CAD build for the part. Positions are in the model's coordinates, mm. Face numbers are marked on the shaded views. A direction names the side the tool comes from. Give positions to 0.01 mm unless a question says otherwise; leave off trailing zeros. Write each loop counter-clockwise with the first axis right and the second up, starting at its lowest first coordinate (ties: lowest second). Pieces come first, ordered by that corner, then holes. Notation, with made-up numbers: (71.25, 51.25) - (75.25, 51.25) arc R13 cw to (75.25, 58.25) - close; hole circle Ø10 at (51.25, -19.5). An arc over 180 degrees is marked (long way). Write item = value, one per line. Start each with the question number.
```python
from build123d import *

# Parameters (mm, degrees)
SKETCH1_W           = 85.95
SKETCH1_H           = 85.95
BOSS_EXTRUDE1_DEPTH = 85.95
SKETCH2_W           = 83.95
SKETCH2_H           = 83.95
CUT_EXTRUDE1_DEPTH  = 83.95
CAVITY1_OUTLINE_R   = 13
CAVITY1_DEPTH       = 2
CAVITY2_OUTLINE_R   = 13
CAVITY2_DEPTH       = 2
CAVITY4_START       = -85.95
CAVITY4_OUTLINE_R   = 13
CAVITY4_DEPTH       = 2
CUT_EXTRUDE3_DEPTH  = 148.724092483
BOSS_EXTRUDE2_DEPTH = 2
CUT_EXTRUDE4_REACH  = 150.87
SKETCH8_W           = 2
SKETCH8_H           = 63.308692683
CUT_EXTRUDE5_REACH  = 150.87
SKETCH9_W           = 67.031257487
SKETCH9_H           = 2
CUT_EXTRUDE6_START  = -2
SKETCH10_W          = 2
SKETCH10_H          = 63.308692683
CUT_EXTRUDE6_DEPTH  = 2


# Read off the part's stored shape, not the designer's step: Cavity1, Cavity2, Cavity4
with BuildPart() as part:
    # Sketch1 → Boss-Extrude1 (new body)
    with BuildSketch(Plane.XY):
        with Locations((42.975, -42.975)):
            Rectangle(SKETCH1_W, SKETCH1_H)
    extrude(amount=BOSS_EXTRUDE1_DEPTH)

    # Sketch2 → Cut-Extrude1 (cut)
    with BuildSketch(Plane(origin=(0, 0, 0), x_dir=(1, 0, 0), z_dir=(0, 1, 0))):
        with Locations((43.975, -43.975)):
            Rectangle(SKETCH2_W, SKETCH2_H)
    extrude(amount=-CUT_EXTRUDE1_DEPTH, mode=Mode.SUBTRACT)

    # Cavity1 outline → Cavity1 (cut)
    with BuildSketch(Plane.XY):
        with Locations((38.75, -47.2)):
            Circle(CAVITY1_OUTLINE_R)
    extrude(amount=CAVITY1_DEPTH, mode=Mode.SUBTRACT)

    # Cavity2 outline → Cavity2 (cut)
    with BuildSketch(Plane.YZ):
        with Locations((-47.2, 39.55)):
            Circle(CAVITY2_OUTLINE_R)
    extrude(amount=CAVITY2_DEPTH, mode=Mode.SUBTRACT)

    # Cavity4 outline → Cavity4 (cut)
    with BuildSketch(Plane(origin=(0, 0, 0), x_dir=(1, 0, 0), z_dir=(0, 1, 0)).offset(CAVITY4_START)):
        with Locations((38.75, -39.55)):
            Circle(CAVITY4_OUTLINE_R)
    extrude(amount=CAVITY4_DEPTH, mode=Mode.SUBTRACT)

    # Sketch4 → Cut-Extrude3 (cut, through all)
    with BuildSketch(Plane.XY.offset(2)):
        Polygon((46.786231243, -31.127537514), (77.913768757, 0), (8.036231243, 0), (30.713768757, -31.127537514), align=None)
        Polygon((54.822462486, -39.163768757), (85.95, -8.036231243), (85.95, -77.939325412), (54.822462486, -55.236231243), align=None)
        Polygon((46.717131732, -63.272462486), (75.06748873, -83.95), (8.036231243, -83.95), (30.713768757, -63.272462486), align=None)
        Polygon((22.677537514, -39.163768757), (2, -10.781462068), (2, -74.090154751), (22.677537514, -55.236231243), align=None)
    cut_extrude3 = extrude(amount=-CUT_EXTRUDE3_DEPTH, mode=Mode.SUBTRACT)

    # Mirror1: Cut-Extrude3 across plane
    add(cut_extrude3.mirror(Plane(origin=(0, -42.975, 42.975), x_dir=(0, 0.7071067811865475, 0.7071067811865477), z_dir=(0, 0.7071067811865476, -0.7071067811865475))), mode=Mode.SUBTRACT)

    # Mirror2: Cut-Extrude3 across plane
    add(cut_extrude3.mirror(Plane(origin=(0, 0, 0), x_dir=(0.7071067811865478, 0, 0.7071067811865472), z_dir=(-0.7071067811865475, 0, 0.7071067811865477))), mode=Mode.SUBTRACT)

    # Sketch6 → Boss-Extrude2 (add)
    with BuildSketch(Plane(origin=(2, 0, 0), x_dir=(0, 0, -1), z_dir=(1, 0, 0))):
        Polygon((-8.036231243, -83.95), (-11.859845249, -83.95), (-34.537382763, -63.272462486), (-30.713768757, -63.272462486), align=None)
    extrude(amount=-BOSS_EXTRUDE2_DEPTH)

    # Cut-Extrude4: up to this face of the body (flat: up to its plane)
    cut_extrude4_end = Plane(part.part.faces().sort_by_distance((18.575077405, -83.95, 13.216062518))[0])
    # Sketch8 → Cut-Extrude4 (cut, up to the picked face)
    with BuildSketch(Plane.XZ.offset(85.95), mode=Mode.PRIVATE) as cut_extrude4_sk1:
        with Locations((1, 43.514191591)):
            Rectangle(SKETCH8_W, SKETCH8_H)
    cut_extrude4_tool1 = split(extrude(cut_extrude4_sk1.sketch, amount=-CUT_EXTRUDE4_REACH, mode=Mode.PRIVATE), bisect_by=cut_extrude4_end, keep=Keep.BOTH, mode=Mode.PRIVATE)
    add(cut_extrude4_tool1.solids().sort_by(Axis((1, -85.95, 43.514192), (0, 1, 0)))[0], mode=Mode.SUBTRACT)

    # Cut-Extrude5: up to this face of the body (flat: up to its plane)
    cut_extrude5_end = Plane(part.part.faces().sort_by_distance((41.551859986, -83.95, 1))[0])
    # Sketch9 → Cut-Extrude5 (cut, up to the picked face)
    with BuildSketch(Plane.XZ.offset(85.95), mode=Mode.PRIVATE) as cut_extrude5_sk1:
        with Locations((41.551859987, 1)):
            Rectangle(SKETCH9_W, SKETCH9_H)
    cut_extrude5_tool1 = split(extrude(cut_extrude5_sk1.sketch, amount=-CUT_EXTRUDE5_REACH, mode=Mode.PRIVATE), bisect_by=cut_extrude5_end, keep=Keep.BOTH, mode=Mode.PRIVATE)
    add(cut_extrude5_tool1.solids().sort_by(Axis((41.55186, -85.95, 1), (0, 1, 0)))[0], mode=Mode.SUBTRACT)

    # Sketch10 → Cut-Extrude6 (cut)
    with BuildSketch(Plane.ZY.offset(CUT_EXTRUDE6_START)):
        with Locations((1, -42.435808409)):
            Rectangle(SKETCH10_W, SKETCH10_H)
    extrude(amount=CUT_EXTRUDE6_DEPTH, mode=Mode.SUBTRACT)


solid = part.part
```
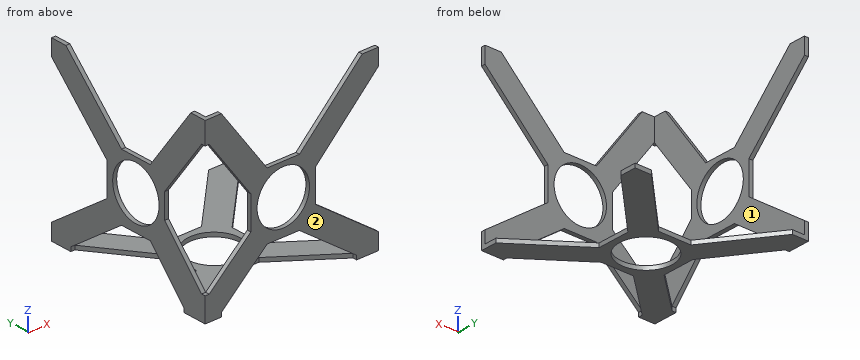
1. Cut at C-C (z = 80). Give the cut face in (x, y), then the cut area to 3 significant figures.
2. Cut at B-B (y = -47.2). Give the cut face in (x, z), then the cut area to 3 significant figures.
3. Pin check, flat tips, straight feed: pin 1 Ø1.6 at (x, z) = (41, 1.5) entering from +Y; pin 2 Ø2 at (x, y) = (49, -29.5) entering from +Z; pin 3 Ø1 at (y, z) = (-84.5, 1.5) entering from -X; pin 4 Ø12 at (y, z) = (-61, 23.5) entering from +X. Stop position of each tip, or through.
4. Wall check: line 1 along Z through (x, y) = (1, -47.2); line 2 along Y through (x, z) = (38.75, 1.5); line 3 along Z through (x, y) = (52, -51). Give the ranges that are in metal, low to high.
5. Cut at A-A (z = 39.55). Give the cut face in (x, y), then the cut area to 3 significant figures.
6. Tool access for the marked faces 1 and 2: list every direction of +Z, -Z, +X, -X, +Y, -Y with a clear straight run to the whole face (end or side of a thin tool).
Output:
q1.outline = (0, -85.95) - (12.37, -85.95) - (12.37, -83.95) - (2, -83.95) - (2, -73.6) - (0, -73.6) - close; (0, -13.99) - (2, -13.99) - (2, 0) - (0, 0) - close; (71.96, -85.95) - (85.95, -85.95) - (85.95, -83.95) - (71.96, -83.95) - close
q1.area = 101 mm2
q2.outline = (0, 22.68) - (2, 22.68) - (2, 26.55) - (0, 26.55) - close; (0, 52.55) - (2, 52.55) - (2, 54.82) - (0, 54.82) - close; (22.68, 0) - (25.75, 0) - (25.75, 2) - (22.68, 2) - close; (51.75, 0) - (54.82, 0) - (54.82, 2) - (51.75, 2) - close
q2.area = 24.6 mm2
q3.pin_1 = -31.13
q3.pin_2 = 2
q3.pin_3 = 0
q3.pin_4 = 2
q4.line_1 = 22.68 to 26.55, 52.55 to 54.82
q4.line_2 = -63.27 to -60.2, -34.2 to -31.13
q4.line_3 = 0 to 2
q5.outline = (0, -63.27) - (2, -63.27) - (2, -60.2) - (0, -60.2) - close; (0, -34.2) - (2, -34.2) - (2, -31.13) - (0, -31.13) - close; (22.68, -85.95) - (25.75, -85.95) - (25.75, -83.95) - (22.68, -83.95) - close; (51.75, -85.95) - (54.82, -85.95) - (54.82, -83.95) - (51.75, -83.95) - close
q5.area = 24.6 mm2
q6.face_1 = +Z, +X, +Y
q6.face_2 = +Z, -Z, +X, -X, -Y
